Build history of the part. All positions in model axes, mm. Face numbers are marked on the shaded views. Give positions to 0.01 mm unless a question says otherwise; leave off trailing zeros. Write each loop counter-clockwise with the first axis right and the second up, starting at its lowest first coordinate (ties: lowest second). Pieces come first, ordered by that corner, then holes. Notation, with made-up numbers: (-24, 23.25) -> (19, 23.25) arc R10 ccw to (19, 33.25) -> close; hole circle Ø4 at (15, 4.25). An arc over 180 degrees is marked (long way). Put each result on its own line as item: value.
Autodesk Inventor part; units mm, degrees
ref_plane "YZ Plane" through (0, 0, 0) normal (1, 0, 0) x (0, 1, 0)
ref_plane "XZ Plane" through (0, 0, 0) normal (0, 1, 0) x (-1, 0, 0)
ref_plane "XY Plane" through (0, 0, 0) normal (0, 0, 1) x (1, 0, 0)
sketch "Sketch1" plane through (0, 0, 0) normal (0, 0, 1) x (1, 0, 0)
  circle A0 centre (0, 0) radius 20
  dimension "d0" = 40
extrude "Extrusion1" add sketch "Sketch1" along normal blind 15
shell "Shell1" thickness 1.5 removed faces 1 at (-2.364, 6.2334, 15)
sketch "Sketch2" plane through (0, 0, 1.5) normal (0, 0, 1) x (1, 0, 0)
  circle A0 centre (0, 0) radius 3
  arc A1 (6, 12.6491) -> (-6, 12.6491) centre (0, 0) ccw construction
  arc A2 (7.5, 15.8114) -> (-7.5, 15.8114) centre (0, 0) ccw
  arc A3 (4.5, 9.4868) -> (-4.5, 9.4868) centre (0, 0) ccw
  arc A4 (4.5, 9.4868) -> (7.5, 15.8114) centre (6, 12.6491) ccw
  arc A5 (-7.5, 15.8114) -> (-4.5, 9.4868) centre (-6, 12.6491) ccw
  line L0 (0, -30.6) -> (0, 43.6)
  dimension "d4" = 6
  dimension "d5" = 7
  dimension "d6" = 14
  dimension "d9" = 12
extrude "Extrusion2" cut sketch "Sketch2" against normal through all
properties part number "principal"
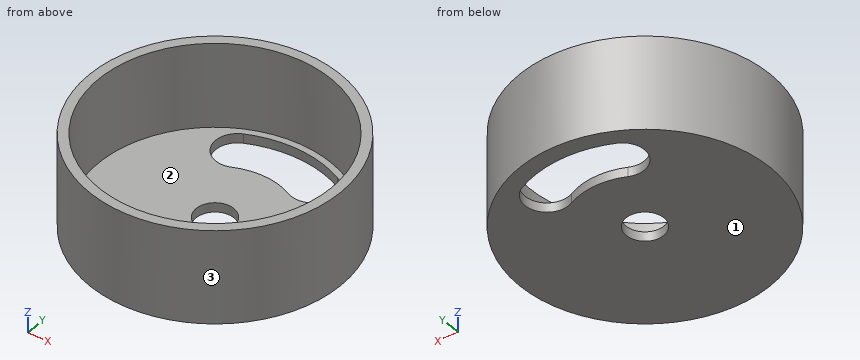
1) Slice it at A-A (x = 0). Write the cut outline in (y, z), plus the area to 3 significant figures.
Filled sheet:
outline: (-20, 0) -> (-3, 0) -> (-3, 1.5) -> (-18.5, 1.5) -> (-18.5, 15) -> (-20, 15) -> close; (3, 0) -> (10.5, 0) -> (10.5, 1.5) -> (3, 1.5) -> close; (17.5, 0) -> (20, 0) -> (20, 15) -> (18.5, 15) -> (18.5, 1.5) -> (17.5, 1.5) -> close
area: 81.0 mm2
2) Pull direction Y, two halves, no side cores. Call the marked faces 1, 2 and 3: released by +Y, released by -Y, zero draft, split by the parting line, or undercut.
Filled sheet:
face 1: zero draft
face 2: undercut
face 3: split by the parting line
3) Wall check: L1, parallel to Y at x = 0, z = 12.75; L2, parallel to Z at x = 3.5, y = 5.5; L3, parallel to Y at x = 12, z = 2.75. Give the ranges that are in metal, low to high.
Filled sheet:
L1: -20 to -18.5, 18.5 to 20
L2: 0 to 1.5
L3: -16 to -14.08, 14.08 to 16
4) Slice it at C-C (x = -6). Write the cut outline in (y, z).
Filled sheet:
outline: (-19.08, 0) -> (9.15, 0) -> (9.15, 1.5) -> (-17.5, 1.5) -> (-17.5, 15) -> (-19.08, 15) -> close; (16.44, 0) -> (19.08, 0) -> (19.08, 15) -> (17.5, 15) -> (17.5, 1.5) -> (16.44, 1.5) -> close
5) Slice it at B-B (y = 0). Write the cut outline in (x, z), plus the area to 3 significant figures.
Filled sheet:
outline: (-20, 0) -> (-3, 0) -> (-3, 1.5) -> (-18.5, 1.5) -> (-18.5, 15) -> (-20, 15) -> close; (3, 0) -> (20, 0) -> (20, 15) -> (18.5, 15) -> (18.5, 1.5) -> (3, 1.5) -> close
area: 91.5 mm2
6) Slice it at D-D (y = 10). Write the cut outline in (x, z), plus the area to 3 significant figures.
Filled sheet:
outline: (-17.32, 0) -> (-8.29, 0) -> (-8.29, 1.5) -> (-15.56, 1.5) -> (-15.56, 15) -> (-17.32, 15) -> close; (-3.2, 0) -> (3.2, 0) -> (3.2, 1.5) -> (-3.2, 1.5) -> close; (8.29, 0) -> (17.32, 0) -> (17.32, 15) -> (15.56, 15) -> (15.56, 1.5) -> (8.29, 1.5) -> close
area: 84.1 mm2
7) Pin check, flat tips, straight feed: pin 1 (1.5 mm diameter, centred on x = 11, y = 5, fed in from +Z); pin 2 (8 mm diameter, centred on x = 15, z = 12.5, fed in from +Y). Stop position of each tip, or through.
Filled sheet:
pin 1: z = 1.5
pin 2: y = 16.7
